```python
from build123d import *

# Parameters (mm, degrees)
SKETCH1_W           = 92
SKETCH1_H           = 44
SKETCH1_R           = 1.090391873
SKETCH1_R_2         = 1.6
SKETCH1_R_3         = 1.26453084
SKETCH1_R_4         = 1.308726881
BOSS_EXTRUDE1_DEPTH = 1.6
FILLET1_R           = 6


with BuildPart() as part:
    # Sketch1 → Boss-Extrude1 (new body)
    with BuildSketch(Plane(origin=(0, 0, 0), x_dir=(1, 0, 0), z_dir=(0, 1, 0))):
        with Locations((46, 22)):
            Rectangle(SKETCH1_W, SKETCH1_H)
        with Locations((2, 6)):
            Circle(SKETCH1_R, mode=Mode.SUBTRACT)
        with Locations((2, 38)):
            Circle(SKETCH1_R_2, mode=Mode.SUBTRACT)
        with Locations((90, 38)):
            Circle(SKETCH1_R_3, mode=Mode.SUBTRACT)
        with Locations((90, 6)):
            Circle(SKETCH1_R_4, mode=Mode.SUBTRACT)
    extrude(amount=BOSS_EXTRUDE1_DEPTH)

    # Fillet1
    fillet1_edges = [part.edges().sort_by_distance(p)[0] for p in [
        (0, 0.8, -44),
        (92, 0.8, -44),
        (92, 0.8, 0),
        (0, 0.8, 0),
    ]]
    fillet(fillet1_edges, radius=FILLET1_R)


solid = part.part
```
Geometry check sheet. Reference: the model listing, model coordinates, mm. Round coordinates to 2 decimals unless told otherwise and drop trailing zeros. Order: outer loops, then holes, each group sorted by start corner. A loop starts at its lowest first (then second) coordinate and runs counter-clockwise, first axis right, second up. Notation, with made-up numbers: (83.5, -13) - (87.5, -13) arc R17 ccw to (87.5, 13) - close; hole circle Ø11 at (-17, -23.75). An arc over 180 degrees is marked (long way). Use a Markdown table: item, result. Add a question column.
1) Gauge pin test, flat ends, axial feed: P1, Ø1.7, axis at x = 2, z = -6, coming from the +Y side; P2, Ø3.5, axis at x = 90, z = -6, coming from the +Y side. Record the tip position at first contact, or that the pin passes through.
2) Mould release check, pull along X, two halves, no side actions. Record for faces 1 (the cylindrical face through (91.17, 0.79, -37.52)), 2 (the flat face through (45, 1, 0)), 3 (the cylindrical face through (1.711, 0.811, -42.196)): released by +X, released by -X, zero draft, split by the parting line, or undercut.
3) Thickness scan on line 1 along X through (y, z) = (0.85, -38); line 2 along X through (y, z) = (1.15, -37); line 3 along Z through (x, y) = (90, 0.85). Record the ranges inside material, lowest first.
4) Section check A-A (x = 90). Record the cut outline in (y, z), then the cut area to 3 significant figures.
5) Section check B-B (x = 2). Record the cut outline in (y, z).
Established:
| question | item | result |
|---|---|---|
| 1 | P1 | through |
| 1 | P2 | y = 1.6 |
| 2 | face 1 | undercut |
| 2 | face 2 | zero draft |
| 2 | face 3 | released by -X |
| 3 | line 1 | 0 to 0.4, 3.6 to 88.74, 91.26 to 92 |
| 3 | line 2 | 0 to 0.75, 3.25 to 89.23, 90.77 to 92 |
| 3 | line 3 | -42.47 to -39.26, -36.74 to -7.31, -4.69 to -1.53 |
| 4 | outline | (0, -42.47) - (1.6, -42.47) - (1.6, -39.26) - (0, -39.26) - close; (0, -36.74) - (1.6, -36.74) - (1.6, -7.31) - (0, -7.31) - close; (0, -4.69) - (1.6, -4.69) - (1.6, -1.53) - (0, -1.53) - close |
| 4 | area | 57.3 mm2 |
| 5 | outline | (0, -42.47) - (1.6, -42.47) - (1.6, -39.6) - (0, -39.6) - close; (0, -36.4) - (1.6, -36.4) - (1.6, -7.09) - (0, -7.09) - close; (0, -4.91) - (1.6, -4.91) - (1.6, -1.53) - (0, -1.53) - close |
